Design review of the part built by this model. Coordinates are the model's own, in mm. Face numbers are marked on the shaded views. A direction names the side the tool comes from. Coordinates: 2 decimals unless noted, no trailing zeros. Loops run counter-clockwise (first coordinate to the right, second up) from the corner with the lowest first, then second, coordinate; pieces in that order, holes last. Notation, with made-up numbers: M 81.25,-10 L 93.25,-10 A19 cw 93.25,27 Z; hole C 15.25,82 d1. An arc over 180 degrees is marked long. Put each result on its own line as item: value. Start each with the question number.
(1) Take a section at B-B, the plane x = 19. Give the boundary of the cut face in (y, z), then the cut area to 3 significant figures.
(2) For the marked faces 1 and 2, list the 3-axis set-ups (+Z, -Z, +X, -X, +Y, -Y) from which the entire face can be reached by the end or side of a thin tool; tool diameter is ignored.
(3) Take a section at D-D, the plane y = -30.5. Give the boundary of the cut face in (x, z), then the cut area to 3 significant figures.
(4) Take a section at C-C, the plane z = -32.5. Give the boundary of the cut face in (x, y).
(5) For probe 1 along Y at (x, z) = (-13, -57); probe 2 along X at (y, z) = (-39.5, -12); probe 3 along X at (y, z) = (-65.25, -53.34), list the stretches that pass through material, from the lowest coordinate up. Write a range as [from, to].
(6) Take a section at A-A, the plane z = -12.7. Give the boundary of the cut face in (x, y), then the cut area to 3 significant figures.
(7) Clearance check with a flat-ended pin moving along its axis: pin 1 (4.5 mm diameter, centred on x = 3.49, z = -53.34, fed in from -Y). State where the tip first meets the part, or that it passes through.
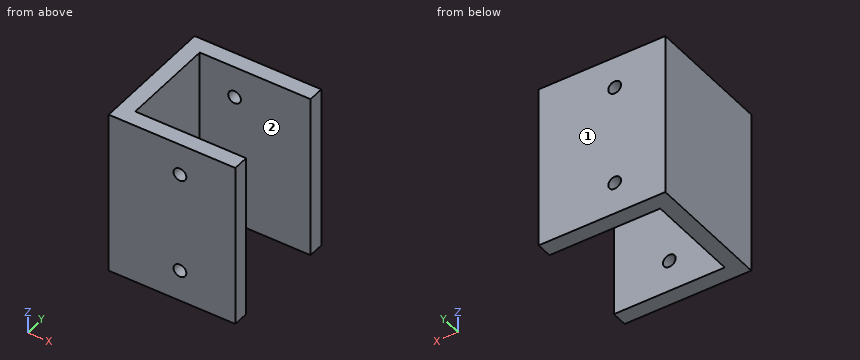
```python
from build123d import *

# Parameters (mm, degrees)
BOSS_EXTRUDE1_DEPTH         = 66.04
F_1_4_20_TAPPED_HOLE1_D     = 5.1054
F_1_4_20_TAPPED_HOLE1_DEPTH = 6.35
F_1_4_20_TAPPED_HOLE2_D     = 5.1054
F_1_4_20_TAPPED_HOLE2_DEPTH = 6.35


with BuildPart() as part:
    # Sketch1 → Boss-Extrude1 (new body)
    with BuildSketch(Plane.XY):
        Polygon((-18.735809365, -25.616936059), (25.714190635, -25.616936059), (25.714190635, -19.266936059), (-25.085809365, -19.266936059), (-25.085809365, -70.066936059), (25.714190635, -70.066936059), (25.714190635, -63.716936059), (-18.735809365, -63.716936059), align=None)
    extrude(amount=-BOSS_EXTRUDE1_DEPTH)

    # 1/4-20 Tapped Hole1
    with Locations(Plane(origin=(0, -19.266936059, 0), x_dir=(1, 0, 0), z_dir=(0, 1, 0))):
        with Locations((-4.765809365, 53.086), (-4.765809365, 12.7)):
            Hole(F_1_4_20_TAPPED_HOLE1_D / 2, depth=F_1_4_20_TAPPED_HOLE1_DEPTH)

    # 1/4-20 Tapped Hole2
    with Locations(Plane(origin=(0, -70.066936059, 0), x_dir=(-1, 0, 0), z_dir=(0, -1, 0))):
        with Locations((-3.489190635, 12.7), (-3.489190635, 53.34)):
            Hole(F_1_4_20_TAPPED_HOLE2_D / 2, depth=F_1_4_20_TAPPED_HOLE2_DEPTH)


solid = part.part
```
Computed values:
1. outline: M -70.07,-66.04 L -63.72,-66.04 L -63.72,0 L -70.07,0 Z; M -25.62,-66.04 L -19.27,-66.04 L -19.27,0 L -25.62,0 Z
1. area: 839 mm^2
2. face 1: +Z, -Z, +X, -X, +Y
2. face 2: +Z, -Z, +X
3. outline: M -25.09,-66.04 L -18.74,-66.04 L -18.74,0 L -25.09,0 Z
3. area: 419 mm^2
4. outline: M -25.09,-70.07 L 25.71,-70.07 L 25.71,-63.72 L -18.74,-63.72 L -18.74,-25.62 L 25.71,-25.62 L 25.71,-19.27 L -25.09,-19.27 Z
5. probe 1: y = [-70.07, -63.72], [-25.62, -19.27]
5. probe 2: x = [-25.09, -18.74]
5. probe 3: x = [-25.09, 0.94], [6.04, 25.71]
6. outline: M -25.09,-70.07 L 0.94,-70.07 L 0.94,-63.72 L -18.74,-63.72 L -18.74,-25.62 L -7.32,-25.62 L -7.32,-19.27 L -25.09,-19.27 Z; M -2.21,-25.62 L 25.71,-25.62 L 25.71,-19.27 L -2.21,-19.27 Z; M 6.04,-70.07 L 25.71,-70.07 L 25.71,-63.72 L 6.04,-63.72 Z
6. area: 822 mm^2
7. pin 1: stops at y = -25.62
